Autodesk Inventor part; units mm, degrees
ref_plane "YZ Plane" through (0, 0, 0) normal (1, 0, 0) x (0, 1, 0)
ref_plane "XZ Plane" through (0, 0, 0) normal (0, 1, 0) x (-1, 0, 0)
ref_plane "XY Plane" through (0, 0, 0) normal (0, 0, 1) x (1, 0, 0)
sketch "Sketch1" plane through (0, 0, 0) normal (0, 0, 1) x (1, 0, 0)
  line L0 (0, -5.5) -> (0, 5.5)
  line L1 (0, 5.5) -> (-0.8, 5.5)
  line L2 (-0.8, 5.5) -> (-0.8, 3.5)
  line L3 (-0.8, 3.5) -> (-2.5, 3.5)
  line L4 (-2.5, 3.5) -> (-2.5, 2)
  line L5 (-2.5, 2) -> (-4, 2)
  line L6 (-4, 2) -> (-4, 1.2)
  line L7 (-4, 1.2) -> (-2.5, 0.8)
  line L8 (-2.5, 0.8) -> (-2.5, -0.8)
  line L9 (-2.5, -0.8) -> (-4, -1.2)
  line L10 (-4, -1.2) -> (-4, -2)
  line L11 (-4, -2) -> (-2.5, -2)
  line L12 (-2.5, -2) -> (-2.5, -3.5)
  line L13 (-2.5, -3.5) -> (-0.8, -3.5)
  line L14 (-0.8, -3.5) -> (-0.8, -5.5)
  line L15 (-0.8, -5.5) -> (0, -5.5)
  point P0 (0, 0)
  point P1 (0, 0)
  point P2 (-2.5, 0)
  dimension "d0" = 11
  dimension "d1" = 5
  dimension "d2" = 1.6
  dimension "d3" = 7
  dimension "d4" = 8
  dimension "d5" = 4
  dimension "d6" = 1.6
  dimension "d7" = 0.8
revolve "Revolution1" add sketch "Sketch1" angle 360 about axis through (0, -5.5, 0) along (0, 1, 0)
properties part number "3464" material "Steel"
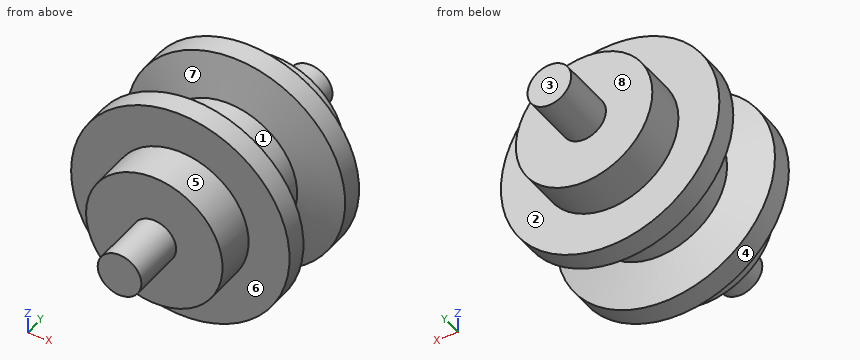
The listing builds one solid part. Answer for the finished solid, in the listing's coordinates (mm). Face numbers are marked on the shaded views. A direction names the side the tool comes from. Round coordinates to 2 decimals unless told otherwise and drop trailing zeros. Order: outer loops, then holes, each group sorted by start corner. A loop starts at its lowest first (then second) coordinate and runs counter-clockwise, first axis right, second up. Notation, with made-up numbers: (-30.5, -35) - (-4.5, -35) arc R10 cw to (-4.5, -29) - close; hole circle Ø7 at (78, 4). An arc over 180 degrees is marked (long way). Write item = value, one per line. Start each with the question number.
1) Section B-B, the plane z = 0 is taken. Write down the section's boundary in (x, y).
2) Given pin 1 (4 mm diameter, centred on x = 1.5, y = 3.5, fed in from +Z); pin 2 (3 mm diameter, centred on x = -2.5, z = -1, fed in from +Y), each flat-ended and moving along its own axis, determine where each tip first touches the part or whether it passes through.
3) Section A-A, the plane x = 0 is taken. Write down the section's boundary in (y, z).
4) For a pull along Y with two mould halves and no side action, classify the marked faces 6, 7 and 8 as released by +Y, released by -Y, zero draft, split by the parting line, or undercut.
5) Section C-C, the plane y = -2.25 is taken. Write down the section's boundary in (x, z).
6) For the marked faces 1, 2, 3, 4 and 5, determine the directions among +Z, -Z, +X, -X, +Y, -Y from which every point of the face is accessible in a straight line to the end or side of a thin tool.
7) Straight lines are drawn through the part: L1, parallel to Z at x = 1.5, y = 0.75; L2, parallel to Y at x = -1.25, z = 1.25; L3, parallel to Y at x = 2.75, z = -1.5. For each, find the intervals that lie inside material, in ascending order.
8) Section D-D, the plane y = 4.5 is taken. Write down the section's boundary in (x, z).
Results list:
q1.outline = (-4, -2) - (-2.5, -2) - (-2.5, -3.5) - (-0.8, -3.5) - (-0.8, -5.5) - (0.8, -5.5) - (0.8, -3.5) - (2.5, -3.5) - (2.5, -2) - (4, -2) - (4, -1.2) - (2.5, -0.8) - (2.5, 0.8) - (4, 1.2) - (4, 2) - (2.5, 2) - (2.5, 3.5) - (0.8, 3.5) - (0.8, 5.5) - (-0.8, 5.5) - (-0.8, 3.5) - (-2.5, 3.5) - (-2.5, 2) - (-4, 2) - (-4, 1.2) - (-2.5, 0.8) - (-2.5, -0.8) - (-4, -1.2) - close
q2.pin_1 = 4
q2.pin_2 = 3.5
q3.outline = (-5.5, -0.8) - (-3.5, -0.8) - (-3.5, -2.5) - (-2, -2.5) - (-2, -4) - (-1.2, -4) - (-0.8, -2.5) - (0.8, -2.5) - (1.2, -4) - (2, -4) - (2, -2.5) - (3.5, -2.5) - (3.5, -0.8) - (5.5, -0.8) - (5.5, 0.8) - (3.5, 0.8) - (3.5, 2.5) - (2, 2.5) - (2, 4) - (1.2, 4) - (0.8, 2.5) - (-0.8, 2.5) - (-1.2, 4) - (-2, 4) - (-2, 2.5) - (-3.5, 2.5) - (-3.5, 0.8) - (-5.5, 0.8) - close
q4.face_6 = released by -Y
q4.face_7 = undercut
q4.face_8 = released by +Y
q5.outline = circle Ø5 at (0, 0)
q6.face_1 = none
q6.face_2 = +Y
q6.face_3 = +Z, -Z, +X, -X, +Y
q6.face_4 = +Y, -Y
q6.face_5 = -Y
q7.L1 = -2 to 2
q7.L2 = -3.5 to 3.5
q7.L3 = -2 to -0.97, 0.97 to 2
q8.outline = circle Ø1.6 at (0, 0)
